Read the model definition and answer for the solid it produces. Units are mm, in the model's axes. A direction names the side the tool comes from. Give positions to 0.01 mm unless a question says otherwise; leave off trailing zeros. Write each loop counter-clockwise with the first axis right and the second up, starting at its lowest first coordinate (ties: lowest second). Pieces come first, ordered by that corner, then holes.
Autodesk Inventor part; units mm, degrees
ref_plane "YZ Plane" through (0, 0, 0) normal (1, 0, 0) x (0, 1, 0)
ref_plane "XZ Plane" through (0, 0, 0) normal (0, 1, 0) x (-1, 0, 0)
ref_plane "XY Plane" through (0, 0, 0) normal (0, 0, 1) x (1, 0, 0)
sketch "Sketch1" plane through (0, 0, 0) normal (1, 0, 0) x (0, 1, 0)
  line L0 (0, 0) -> (1.6002, 0)
  line L1 (1.6002, 0) -> (1.6002, -12.7)
  line L2 (1.6002, -12.7) -> (0, -12.7)
  line L3 (0, -12.7) -> (0, 0)
  line L4 (0, -12.7) -> (0, -11.0998)
  line L5 (0, -11.0998) -> (12.7, -11.0998)
  line L6 (12.7, -11.0998) -> (12.7, -12.7)
  line L7 (12.7, -12.7) -> (0, -12.7)
  line L8 (0, -12.7) -> (0, -11.0998)
  point P0 (1.6002, -11.0998)
  dimension "d0" = 1.6002
  dimension "d1" = 12.7
  dimension "d2" = 1.6002
  dimension "d3" = 12.7
extrude "Extrusion1" add sketch "Sketch1" along normal blind 152.4
sketch "Sketch4" plane through (0, 0, 0) normal (0, 0, 1) x (1, 0, 0)
  line L0 (0, 1.6002) -> (152.4, 1.6002)
  line L1 (0, 0) -> (152.4, 0)
  line L2 (152.4, 0) -> (152.4, 1.6002)
  line L3 (152.4, 1.6002) -> (0, 1.6002)
  line L4 (0, 1.6002) -> (0, 0)
extrude "Extrusion4" add sketch "Sketch4" along normal blind 6.35
sketch "Sketch5" plane through (0, 12.7, -11.0998) normal (0, 1, 0) x (1, 0, 0)
  line L0 (0, 0) -> (152.4, 0)
  line L1 (152.4, 1.6002) -> (152.4, -17.4498)
  line L2 (0, 0) -> (152.4, 0)
  line L3 (152.4, 0) -> (152.4, 1.6002)
  line L4 (152.4, 1.6002) -> (0, 1.6002)
  line L5 (0, 1.6002) -> (0, 0)
  point P0 (0, -11.0998)
extrude "Extrusion5" add sketch "Sketch5" along normal blind 6.35
sketch "Sketch6" plane through (0, 1.6002, -11.0998) normal (0, 1, 0) x (1, 0, 0)
  point P0 (0, -11.0998)
sketch "Sketch7" plane through (0, 1.6002, -11.0998) normal (0, 1, 0) x (1, 0, 0)
  line L0 (152.4, 1.6002) -> (152.4, -17.4498)
  line L1 (152.4, -17.4498) -> (152.4, 0.0127)
  line L2 (152.4, -8.7185) -> (146.8374, -8.7185)
  line L3 (146.8374, -8.7185) -> (121.4374, -8.7185)
  circle A0 centre (121.4374, -8.7185) radius 2.1082
  line L4 (121.4374, -8.7185) -> (73.1774, -8.7186)
  circle A1 centre (73.1774, -8.7186) radius 2.1082
  line L5 (146.8374, -8.7185) -> (146.8374, -4.9085)
  circle A2 centre (146.8374, -4.9085) radius 2.1082
  point P0 (0, -11.0998)
  dimension "d19" = 17.4625
  dimension "d20" = 5.5626
  dimension "d22" = 25.4
  dimension "d23" = 48.26
  dimension "d24" = 4.2164
  dimension "d27" = 3.81
  dimension "d28" = 4.2164
extrude "Extrusion6" cut sketch "Sketch7" against normal blind 25.4
properties part number "wing"
Item 1: Determine the mould class of faces 3 (the cylindrical face through (148.785, 0.811, -5.384)), 4 (the flat face through (77, 9, -12.7)), 5 (the flat face through (152.4, 5, -12)) for opening direction Z: pulls with the +Z half, pulls with the -Z half, needs draft (parallel to the pull), parting line crosses it, or undercut.
Result set:
face 3: undercut
face 4: pulls with the -Z half
face 5: needs draft
Item 2: Section A-A (x = 55) is taken. Write down the section's boundary in (y, z), and give its area (3 significant figures).
Result set:
outline: (0, -12.7) - (19.05, -12.7) - (19.05, -11.1) - (1.6, -11.1) - (1.6, 6.35) - (0, 6.35) - close
area: 58.4 mm2
Item 3: Section B-B (z = 4) is taken. Write down the section's boundary in (x, y), and give its area (3 significant figures).
Result set:
outline: (0, 0) - (152.4, 0) - (152.4, 1.6) - (0, 1.6) - close
area: 244 mm2
Item 4: Find the intervals of material crossed by line 1 along X through (y, z) = (1.5, -0.75); line 2 along Z through (x, y) = (38, 17.25); line 3 along Y through (x, z) = (125.5, -4.5), in increasing order.
Result set:
line 1: x = 0 to 71.84, 74.51 to 120.1, 122.77 to 152.4
line 2: z = -12.7 to -11.1
line 3: y = 0 to 1.6
Item 5: Each of these flat-tipped pins is pushed along its axis until it touches: pin 1 Ø10 at (x, y) = (16, 17) entering from +Z; pin 2 Ø8 at (y, z) = (11, -3.5) entering from -X. Where does it stop, or does it pass through?
Result set:
pin 1: stops at z = -11.1
pin 2: passes through
Item 6: Section C-C (y = 11.5) is taken. Write down the section's boundary in (x, z).
Result set:
outline: (0, -12.7) - (152.4, -12.7) - (152.4, -11.1) - (0, -11.1) - close
Item 7: Which of the six approach directions +Z, -Z, +X, -X, +Y, -Y give full straight-line access (tool end or side, diameter ignored) to faces 1 (the flat face through (75, 1.6, -4)), 2 (the flat face through (75, 0, -1))?
Result set:
face 1: +Z, +X, -X, +Y
face 2: +Z, -Z, +X, -X, -Y
